Can you work these out from the drawing? Everything is in mm from the part's minimum corner. A direction names the side the tool comes from. Give positions to 0.01 mm unless a question says otherwise; leave off trailing zeros. Loops run counter-clockwise (first coordinate to the right, second up) from the corner with the lowest first, then second, coordinate; pieces in that order, holes last.
Q1. If we section it at D-D (x = 12): Please give me the cut outline in (y, z).
Q2. If we section it at B-B (y = 68): Please give me the cut outline in (x, z).
Q3. For the marked faces 4 and 5, which set-ups out of +Z, -Z, +X, -X, +Y, -Y let a thin tool reach every point of the face, with its end or its side?
Q4. We'd pull the mould along X, two halves only. Please class the marked faces 1, 2 and 3: +X half, -X half, draft (parallel to the pull), parting line (faces both ways), or undercut.
Q5. If we section it at A-A (z = 85.5): Please give me the cut outline in (x, y).
Q6. Will these pins go through, and if not, where does the flat tip stop? P1, Ø1.6, axis at x = 41.5, z = 99.5, coming from the +Y side; P2, Ø1.5, axis at x = 13, y = 62.5, coming from the -Z side; P3, Ø0.9, axis at x = 1, z = 65, coming from the +Y side.
Q7. I need wall thicknesses on line 1 (X direction, y = 22, z = 41.5); line 2 (Z direction, x = 29, y = 23.5). Which ranges of each line are inside material? Lowest first, please.
Q8. If we section it at C-C (y = 26.5): Please give me the cut outline in (x, z).
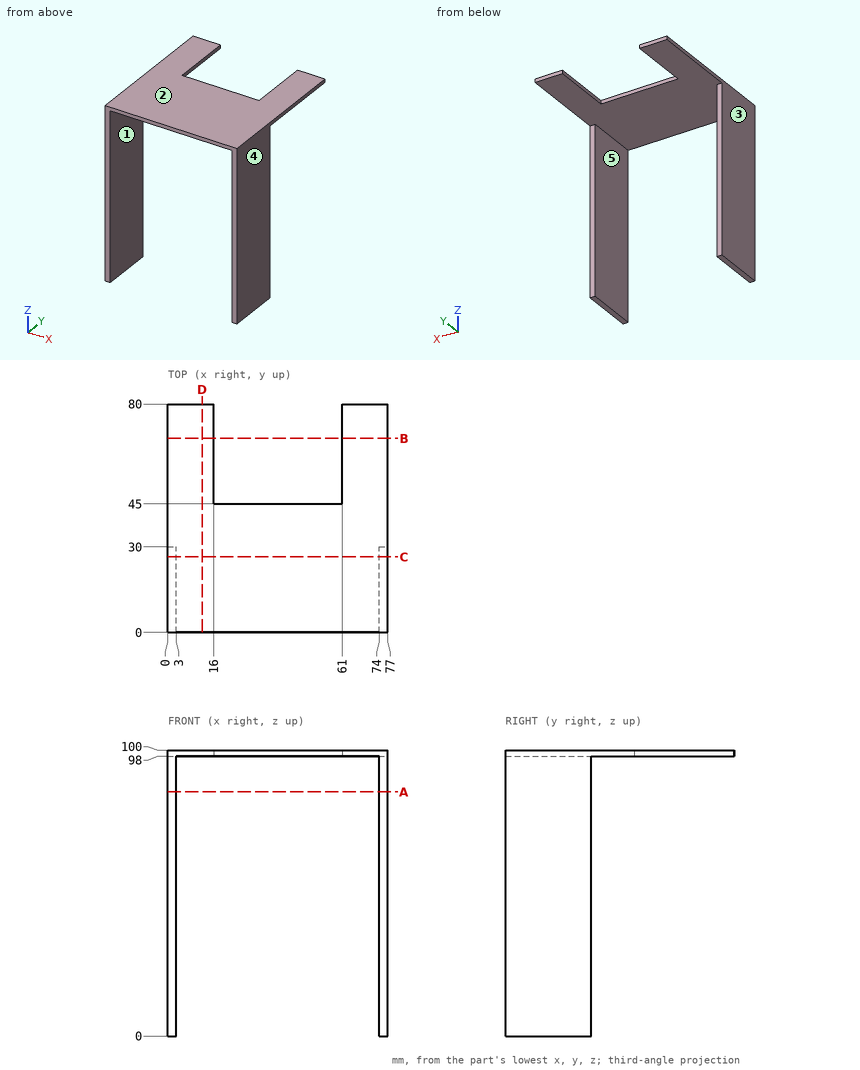
Check sheet entries:
1. outline: (0, 98) - (80, 98) - (80, 100) - (0, 100) - close
2. outline: (0, 98) - (16, 98) - (16, 100) - (0, 100) - close; (61, 98) - (77, 98) - (77, 100) - (61, 100) - close
3. face 4: +Z, -Z, +X, +Y, -Y
3. face 5: -Z, +Y, -Y
4. face 1: undercut
4. face 2: draft
4. face 3: -X half
5. outline: (0, 0) - (3, 0) - (3, 30) - (0, 30) - close; (74, 0) - (77, 0) - (77, 30) - (74, 30) - close
6. P1: stops at y = 45
6. P2: stops at z = 98
6. P3: stops at y = 30
7. line 1: x = 0 to 3, 74 to 77
7. line 2: z = 98 to 100
8. outline: (0, 0) - (3, 0) - (3, 98) - (74, 98) - (74, 0) - (77, 0) - (77, 100) - (0, 100) - close
